Model file for the job. Use its own axes, mm. A direction names the side the tool comes from. Coordinates: 2 decimals unless noted, no trailing zeros. Order: outer loops, then holes, each group sorted by start corner. A loop starts at its lowest first (then second) coordinate and runs counter-clockwise, first axis right, second up. Notation, with made-up numbers: (52.25, 84.25) - (58.25, 84.25) arc R21 cw to (58.25, 92.25) - close; hole circle Ø5 at (20.5, -34.5). An arc over 180 degrees is marked (long way). Put each result on its own line as item: value. Start each with the question number.
```python
from build123d import *

# Parameters (mm, degrees)
SKETCH1_R                    = 12.7
MOUNTING_FLANGE_DEPTH        = 6
SKETCH3_R                    = 6.35
MOTOR_SHAFT_RELIEF_DEPTH     = 2.54
SKETCH2_R                    = 2.5
DRIVE_SHAFT_DEPTH            = 17.272
CHAMFER1_SIZE                = 0.508
SKETCH5_R                    = 4.7625
SHAFT_SUPPORT_SHOULDER_DEPTH = 7.62
M2_5_CLEARANCE_HOLE_D        = 2.9
SKETCH8_R                    = 2.38125
M2_5_TIGHT_COUTERBORE_DEPTH  = 3.048
CIRPATTERN_COUNT             = 3


with BuildPart() as part:
    # Sketch1 → Mounting Flange (new body)
    with BuildSketch(Plane.XY):
        Circle(SKETCH1_R)
    extrude(amount=MOUNTING_FLANGE_DEPTH)

    # Sketch3 → Motor Shaft Relief (cut)
    with BuildSketch(Plane(origin=(0, 0, 0), x_dir=(-1, 0, 0), z_dir=(0, 0, -1))):
        Circle(SKETCH3_R)
    extrude(amount=-MOTOR_SHAFT_RELIEF_DEPTH, mode=Mode.SUBTRACT)

    # Sketch2 → Drive Shaft (add)
    with BuildSketch(Plane.XY.offset(6)):
        Circle(SKETCH2_R)
    extrude(amount=DRIVE_SHAFT_DEPTH)

    # Chamfer1
    chamfer1_edges = [part.edges().sort_by_distance(p)[0] for p in [
        (-2.5, 0, 23.272),
    ]]
    chamfer(chamfer1_edges, length=CHAMFER1_SIZE)

    # Sketch5 → Shaft Support Shoulder (add)
    with BuildSketch(Plane.XY.offset(6)):
        with Locations(Location((0, 0, 0), (0, 0, 180))):
            Circle(SKETCH5_R)
    extrude(amount=SHAFT_SUPPORT_SHOULDER_DEPTH)

    # M2.5 Clearance Hole (through all)
    with Locations(Plane.XY.offset(6)):
        with Locations((0, 7.5)):
            m2_5_clearance_hole = Hole(M2_5_CLEARANCE_HOLE_D / 2)

    # Sketch8 → M2.5 Tight Couterbore (cut)
    with BuildSketch(Plane.XY.offset(6)):
        with Locations((0, 7.5)):
            Circle(SKETCH8_R)
    m2_5_tight_couterbore = extrude(amount=-M2_5_TIGHT_COUTERBORE_DEPTH, mode=Mode.SUBTRACT)

    # CirPattern: M2.5 Clearance Hole, M2.5 Tight Couterbore ×3 about axis
    cirpattern_axis = Axis((0, 0, 0), (0, 0, 1))
    add([m2_5_clearance_hole.rotate(cirpattern_axis, i * 360 / CIRPATTERN_COUNT) for i in range(1, CIRPATTERN_COUNT)], mode=Mode.SUBTRACT)
    add([m2_5_tight_couterbore.rotate(cirpattern_axis, i * 360 / CIRPATTERN_COUNT) for i in range(1, CIRPATTERN_COUNT)], mode=Mode.SUBTRACT)


solid = part.part
```
Item 1: 3-axis set-ups, long thin cutter, end or side, ignore diameter. For faces 1 (the face through (0, 0, 23.272)), 2 (the face through (6, -2, 2.952)), 3 (the face through (-5.54, 3.1, 1.25)): which of +Z, -Z, +X, -X, +Y, -Y reach the whole face in a straight line?
Item 2: Slice it at D-D, the plane z = 21.75. Give the cut face in (x, y).
Item 3: Slice it at C-C, the plane y = 0. Give the cut face in (x, z), plus the area to 3 significant figures.
Item 4: Wall check: line 1 along Y through (x, z) = (0, 1.5); line 2 along Y through (x, z) = (0, 4.45); line 3 along X through (y, z) = (-3.75, 0.75). Give the ranges that are in metal, low to high.
Item 5: Flat gauge pins, fed straight in: pin 1 Ø4.5 at (x, y) = (0, 7.5) entering from +Z; pin 2 Ø10 at (x, y) = (3, 10) entering from +Z; pin 3 Ø10 at (x, z) = (-6.5, 13) entering from -Y. Where does each tip first touch, or does it go through?
Item 6: Slice it at B-B, the plane y = 7.5. Give the cut face in (x, z).
Item 7: Pull direction X, two halves, no side cores. Call faces 4 (the face through (1.03, 4.65, 9.76)), 5 (the face through (-4.224, -3.035, 4.497)), 6 (the face through (3, 6, 0)): pulls with the +X half, pulls with the -X half, needs draft (parallel to the pull), parting line crosses it, or undercut.
Item 8: Slice it at A-A, the plane x = 0. Give the cut face in (y, z).
Here are the results:
1. face 1: +Z, +X, -X, +Y, -Y
1. face 2: +Z
1. face 3: -Z
2. outline: circle Ø5 at (0, 0)
3. outline: (-12.7, 0) - (-6.35, 0) - (-6.35, 2.54) - (6.35, 2.54) - (6.35, 0) - (12.7, 0) - (12.7, 6) - (4.76, 6) - (4.76, 13.62) - (2.5, 13.62) - (2.5, 22.76) - (1.99, 23.27) - (-1.99, 23.27) - (-2.5, 22.76) - (-2.5, 13.62) - (-4.76, 13.62) - (-4.76, 6) - (-12.7, 6) - close
3. area: 241 mm^2
4. line 1: y = -12.7 to -6.35, 8.95 to 12.7
4. line 2: y = -12.7 to 5.12, 9.88 to 12.7
4. line 3: x = -12.13 to -7.95, 7.95 to 12.13
5. pin 1: stops at z = 2.95
5. pin 2: stops at z = 6
5. pin 3: stops at y = -4.52
6. outline: (-10.25, 0) - (-1.45, 0) - (-1.45, 2.95) - (-2.38, 2.95) - (-2.38, 6) - (-10.25, 6) - close; (1.45, 0) - (10.25, 0) - (10.25, 6) - (2.38, 6) - (2.38, 2.95) - (1.45, 2.95) - close
7. face 4: parting line crosses it
7. face 5: undercut
7. face 6: needs draft
8. outline: (-12.7, 0) - (-6.35, 0) - (-6.35, 2.54) - (6.05, 2.54) - (6.05, 2.95) - (5.12, 2.95) - (5.12, 6) - (4.76, 6) - (4.76, 13.62) - (2.5, 13.62) - (2.5, 22.76) - (1.99, 23.27) - (-1.99, 23.27) - (-2.5, 22.76) - (-2.5, 13.62) - (-4.76, 13.62) - (-4.76, 6) - (-12.7, 6) - close; (8.95, 0) - (12.7, 0) - (12.7, 6) - (9.88, 6) - (9.88, 2.95) - (8.95, 2.95) - close
